from build123d import *

# Parameters (mm, degrees)
BOSS_EXTRUDE1_DEPTH  = 5
M5_CLEARANCE_HOLE1_D = 5.5
FILLET1_R            = 5
FILLET2_R            = 0.5


with BuildPart() as part:
    # Sketch1 → Boss-Extrude1 (new body)
    with BuildSketch(Plane(origin=(0, 0, 0), x_dir=(1, 0, 0), z_dir=(0, 1, 0))):
        Polygon((-118.5, 0), (118.5, 0), (118.5, 45), (101, 45), (101, 36.5), (31, 36.5), (31, 46.5), (-31, 46.5), (-31, 36.5), (-101, 36.5), (-101, 45), (-118.5, 45), align=None)
    extrude(amount=-BOSS_EXTRUDE1_DEPTH)

    # M5 Clearance Hole1 (through all)
    with Locations(Plane(origin=(0, 0, 0), x_dir=(1, 0, 0), z_dir=(0, 1, 0))):
        with Locations((-111, 37.5), (-111, 17.5), (111, 37.5), (111, 17.5)):
            Hole(M5_CLEARANCE_HOLE1_D / 2)

    # Fillet1
    fillet1_edges = [part.edges().sort_by_distance(p)[0] for p in [
        (-118.5, -2.5, -45),
        (118.5, -2.5, -45),
        (118.5, -2.5, 0),
        (-118.5, -2.5, 0),
    ]]
    fillet(fillet1_edges, radius=FILLET1_R)

    # Fillet2
    fillet2_edges = [part.edges().sort_by_distance(p)[0] for p in [
        (-101, -2.5, -45),
        (-101, -2.5, -36.5),
        (-31, -2.5, -36.5),
        (-31, -2.5, -46.5),
        (31, -2.5, -46.5),
        (31, -2.5, -36.5),
        (101, -2.5, -36.5),
        (101, -2.5, -45),
    ]]
    fillet(fillet2_edges, radius=FILLET2_R)


solid = part.part
The listing builds one solid part. Answer for the finished solid, in the listing's coordinates (mm). A direction names the side the tool comes from. Coordinates: 2 decimals unless noted, no trailing zeros. Loops run counter-clockwise (first coordinate to the right, second up) from the corner with the lowest first, then second, coordinate; pieces in that order, holes last.
1) A tool of negligible diameter and unlimited length cuts with its end or side. For faces 1 (the face through (108, -2, -45)), 2 (the face through (-66, -2, -36.5)), 3 (the face through (113.027, -2.535, -39.359)), 4 (the face through (-107, -2, -45)), from which of +Z, -Z, +X, -X, +Y, -Y can it reach the whole face along a straight path? Write none if from no direction.
2) Find section D-D on x = 95. Write down the section's boundary in (y, z).
3) Find section A-A on y = -2.3. Write down the section's boundary in (x, z), then the cut area to 3 significant figures.
4) Find section C-C on z = -17.5. Write down the section's boundary in (x, y), then the cut area to 3 significant figures.
5) Find the intervals of material crossed by L1, parallel to Z at x = 111, y = -3.05; L2, parallel to X at y = -0.3, z = -18; L3, parallel to X at y = -4.4, z = -41, in increasing order.
6) Flat-ended cylindrical pins translate along their axes: pin 1 Ø4.5 at (x, z) = (-111, -17.5) entering from +Y; pin 2 Ø2.5 at (x, y) = (-108, -3) entering from -Z. Find the tip coordinate at first contact, or state that the pin passes through.
7) Find section B-B on x = -111. Write down the section's boundary in (y, z).
8) Determine the mould class of faces 5 (the face through (-101, -2, -41)), 6 (the face through (66, -2, -36.5)), 7 (the face through (117.07, -2.54, -43.5)), 8 (the face through (-117.07, -2.54, -43.5)) for opening direction X: pulls with the +X half, pulls with the -X half, needs draft (parallel to the pull), parting line crosses it, or undercut.
Values:
1. face 1: -Z, +X, +Y, -Y
1. face 2: -Z, +Y, -Y
1. face 3: +Y, -Y
1. face 4: -Z, -X, +Y, -Y
2. outline: (-5, -36.5) - (0, -36.5) - (0, 0) - (-5, 0) - close
3. outline: (-118.5, -40) arc R5 ccw to (-113.5, -45) - (-101.5, -45) arc R0.5 ccw to (-101, -44.5) - (-101, -37) arc R0.5 cw to (-100.5, -36.5) - (-31.5, -36.5) arc R0.5 cw to (-31, -37) - (-31, -46) arc R0.5 ccw to (-30.5, -46.5) - (30.5, -46.5) arc R0.5 ccw to (31, -46) - (31, -37) arc R0.5 cw to (31.5, -36.5) - (100.5, -36.5) arc R0.5 cw to (101, -37) - (101, -44.5) arc R0.5 ccw to (101.5, -45) - (113.5, -45) arc R5 ccw to (118.5, -40) - (118.5, -5) arc R5 ccw to (113.5, 0) - (-113.5, 0) arc R5 ccw to (-118.5, -5) - close; hole circle Ø5.5 at (-111, -37.5); hole circle Ø5.5 at (-111, -17.5); hole circle Ø5.5 at (111, -37.5); hole circle Ø5.5 at (111, -17.5)
3. area: 9,450 mm2
4. outline: (-118.5, -5) - (-113.75, -5) - (-113.75, 0) - (-118.5, 0) - close; (-108.25, -5) - (108.25, -5) - (108.25, 0) - (-108.25, 0) - close; (113.75, -5) - (118.5, -5) - (118.5, 0) - (113.75, 0) - close
4. area: 1,130 mm2
5. L1: z = -45 to -40.25, -34.75 to -20.25, -14.75 to 0
5. L2: x = -118.5 to -113.7, -108.3 to 108.3, 113.7 to 118.5
5. L3: x = -118.4 to -101, -31 to 31, 101 to 118.4
6. pin 1: passes through
6. pin 2: stops at z = -45
7. outline: (-5, -45) - (0, -45) - (0, -40.25) - (-5, -40.25) - close; (-5, -34.75) - (0, -34.75) - (0, -20.25) - (-5, -20.25) - close; (-5, -14.75) - (0, -14.75) - (0, 0) - (-5, 0) - close
8. face 5: undercut
8. face 6: undercut
8. face 7: pulls with the +X half
8. face 8: pulls with the -X half
